Geometry check sheet. Reference: the model listing, model coordinates, mm. A direction names the side the tool comes from. Give positions to 0.01 mm unless a question says otherwise; leave off trailing zeros. Order: outer loops, then holes, each group sorted by start corner. A loop starts at its lowest first (then second) coordinate and runs counter-clockwise, first axis right, second up. Notation, with made-up numbers: M 57,33 L 94,33 A21 cw 94,56 Z; hole C -7,77.5 d11. An arc over 180 degrees is marked long. Answer as CSV lines item,"result". Start each with the question number.
```python
from build123d import *

# Parameters (mm, degrees)
RESSALTO_EXTRUS_O3_DEPTH   = 89
FILETE3_R                  = 1
ESBO_O16_W                 = 12
ESBO_O16_H                 = 1
RESSALTO_EXTRUS_O5_DEPTH   = 0.5
FILETE7_R                  = 0.5
CORTE_EXTRUS_O9_DEPTH      = 200
CORTE_EXTRUS_O9_DEPTH_BACK = 10
ESBO_O22_R                 = 1.25
ESBO_O22_W                 = 8
ESBO_O22_H                 = 15
CORTE_EXTRUS_O10_DEPTH     = 322.757399842
RESSALTO_EXTRUS_O8_DEPTH   = 2
FILETE12_R                 = 10
FILETE13_R                 = 4
ESBO_O30_W                 = 10
ESBO_O30_H                 = 1.5
RESSALTO_EXTRUS_O10_DEPTH  = 0.75
FILETE14_R                 = 0.75
RESSALTO_EXTRUS_O11_START  = -20
RESSALTO_EXTRUS_O11_DEPTH  = 5


with BuildPart() as part:
    # Esboço6 → Ressalto-extrusão3 (new body)
    with BuildSketch(Plane(origin=(0, -284.347629413, 0), x_dir=(1, 0, 0), z_dir=(0, 1, 0))):
        Polygon((4.5, 12.61291239), (2.5, 12.61291239), (2.5, 32.61291239), (149.5, 32.61291239), (149.5, 12.61291239), (147.5, 12.61291239), (147.5, 30.61291239), (4.5, 30.61291239), align=None)
    extrude(amount=RESSALTO_EXTRUS_O3_DEPTH)

    # Filete3
    filete3_edges = [part.edges().sort_by_distance(p)[0] for p in [
        (2.5, -239.847629413, -32.61291239),
        (149.5, -239.847629413, -32.61291239),
    ]]
    fillet(filete3_edges, radius=FILETE3_R)

    # Esboço16 → Ressalto-extrusão5 (add)
    with BuildSketch(Plane.XY.offset(-30.61291239)):
        with Locations((62, -266.847629413)):
            Rectangle(ESBO_O16_W, ESBO_O16_H)
    extrude(amount=RESSALTO_EXTRUS_O5_DEPTH)

    # Filete7
    filete7_edges = [part.edges().sort_by_distance(p)[0] for p in [
        (56, -266.847629413, -30.61291239),
        (68, -266.847629413, -30.61291239),
        (62, -266.347629413, -30.61291239),
        (62, -267.347629413, -30.61291239),
    ]]
    fillet(filete7_edges, radius=FILETE7_R - 0.0001)  # a hair under: the kernel refuses the full size

    # Esboço20 → Corte-extrusão9 (cut, two sides: drawn at the far end of the back side and taken through both)
    with BuildSketch(Plane.ZY.offset(-147.5).offset(-CORTE_EXTRUS_O9_DEPTH_BACK)):
        Polygon((-27.61291239, -195.347629413), (-12.61291239, -195.347629413), (-12.61291239, -248.347629413), align=None)
        with BuildLine():
            Line((-19.964933879, -248.075306948), (-24.796932275, -231.002245945))
            ThreePointArc((-24.796932275, -231.002245945), (-25.896604597, -230.284061963), (-26.759138321, -231.274568411))
            Line((-26.759138321, -231.274568411), (-26.759138321, -248.347629413))
            ThreePointArc((-26.759138321, -248.347629413), (-26.466245102, -249.054736195), (-25.759138321, -249.347629413))
            Line((-25.759138321, -249.347629413), (-20.927139924, -249.347629413))
            ThreePointArc((-20.927139924, -249.347629413), (-20.129542762, -248.950819903), (-19.964933879, -248.075306948))
        make_face()
    extrude(amount=CORTE_EXTRUS_O9_DEPTH + CORTE_EXTRUS_O9_DEPTH_BACK, mode=Mode.SUBTRACT)

    # Esboço22 → Corte-extrusão10 (cut, through all)
    with BuildSketch(Plane.XY.offset(-30.61291239)):
        with Locations((16.25, -277.347629413)):
            Circle(ESBO_O22_R)
        with Locations((135.75, -277.347629413)):
            Circle(ESBO_O22_R)
        with BuildLine():
            Line((131.970562748, -195.347629413), (20.029437252, -195.347629413))
            Line((20.029437252, -195.347629413), (67.514718626, -242.832910788))
            ThreePointArc((67.514718626, -242.832910788), (76, -246.347629413), (84.485281374, -242.832910788))
            Line((84.485281374, -242.832910788), (131.970562748, -195.347629413))
        make_face()
        with BuildLine():
            Line((134.5, -223.688249847), (134.5, -242.347629413))
            ThreePointArc((134.5, -242.347629413), (133.328427125, -245.176056538), (130.5, -246.347629413))
            Line((130.5, -246.347629413), (111.840620434, -246.347629413))
            ThreePointArc((111.840620434, -246.347629413), (108.145102304, -243.878363143), (109.012193309, -239.519202289))
            Line((109.012193309, -239.519202289), (127.671572875, -220.859822722))
            ThreePointArc((127.671572875, -220.859822722), (132.030733729, -219.992731717), (134.5, -223.688249847))
        make_face()
        with BuildLine():
            Line((17.5, -223.688249847), (17.5, -242.347629413))
            ThreePointArc((17.5, -242.347629413), (18.671572875, -245.176056538), (21.5, -246.347629413))
            Line((21.5, -246.347629413), (40.159379566, -246.347629413))
            ThreePointArc((40.159379566, -246.347629413), (43.854897696, -243.878363143), (42.987806691, -239.519202289))
            Line((42.987806691, -239.519202289), (24.328427125, -220.859822722))
            ThreePointArc((24.328427125, -220.859822722), (19.969266271, -219.992731717), (17.5, -223.688249847))
        make_face()
        with Locations((62, -276.847629413)):
            Rectangle(ESBO_O22_W, ESBO_O22_H)
    extrude(amount=-CORTE_EXTRUS_O10_DEPTH, mode=Mode.SUBTRACT)

    # Esboço25 → Ressalto-extrusão8 (add)
    with BuildSketch(Plane(origin=(0, -195.347629413, 0), x_dir=(1, 0, 0), z_dir=(0, 1, 0))):
        Polygon((147.5, 30.61291239), (142.5, 30.61291239), (147.5, 27.61291239), align=None)
        Polygon((4.5, 30.61291239), (9.5, 30.61291239), (4.5, 27.61291239), align=None)
    extrude(amount=-RESSALTO_EXTRUS_O8_DEPTH)

    # Filete12
    filete12_edges = [part.edges().sort_by_distance(p)[0] for p in [
        (20.029437252, -195.347629413, -31.61291239),
        (131.970562748, -195.347629413, -31.61291239),
    ]]
    fillet(filete12_edges, radius=FILETE12_R)

    # Filete13
    filete13_edges = [part.edges().sort_by_distance(p)[0] for p in [
        (58, -269.347629413, -31.61291239),
        (66, -269.347629413, -31.61291239),
    ]]
    fillet(filete13_edges, radius=FILETE13_R - 0.0001)  # a hair under: the kernel refuses the full size

    # Esboço30 → Ressalto-extrusão10 (add)
    with BuildSketch(Plane.XY.offset(-30.61291239)):
        with Locations((91.5, -258.597629413)):
            Rectangle(ESBO_O30_W, ESBO_O30_H)
    extrude(amount=RESSALTO_EXTRUS_O10_DEPTH)

    # Filete14
    filete14_edges = [part.edges().sort_by_distance(p)[0] for p in [
        (91.5, -257.847629413, -29.86291239),
        (91.5, -259.347629413, -29.86291239),
    ]]
    fillet(filete14_edges, radius=FILETE14_R - 0.0001)  # a hair under: the kernel refuses the full size

    # Esboço31 → Ressalto-extrusão11 (add)
    with BuildSketch(Plane.XZ.offset(284.347629413).offset(RESSALTO_EXTRUS_O11_START)):
        with BuildLine():
            Line((147.5, -30.61291239), (142.5, -30.61291239))
            ThreePointArc((142.5, -30.61291239), (146.035533906, -29.148446296), (147.5, -25.61291239))
            Line((147.5, -25.61291239), (147.5, -30.61291239))
        make_face()
        with BuildLine():
            Line((4.5, -30.61291239), (9.5, -30.61291239))
            ThreePointArc((9.5, -30.61291239), (5.964466094, -29.148446296), (4.5, -25.61291239))
            Line((4.5, -25.61291239), (4.5, -30.61291239))
        make_face()
    extrude(amount=-RESSALTO_EXTRUS_O11_DEPTH)


solid = part.part
```
Item 1: Depth check by flat-ended pin: pin 1 Ø1 at (x, y) = (148.5, -240.5) entering from +Z; pin 2 Ø2.5 at (x, z) = (7.5, -29) entering from -Y; pin 3 Ø0.6 at (x, z) = (123, -32) entering from +Y. Enter the tip coordinate at first touch or a pass-through.
Item 2: Section check B-B on z = -23.25. Record the boundary of the cut face in (x, y), then the cut area to 3 significant figures.
Item 3: Scan lines: line 1 along X through (y, z) = (-248.5, -18.25); line 2 along Y through (x, z) = (135.75, -31.4); line 3 along X through (y, z) = (-237.5, -31). Record each from-to range of solid material in increasing order.
Item 4: Draft check along X on faces 4 (the face through (148.514, -239.658, -22.347)), 5 (the face through (4.5, -250, -22)). Enter one of: pulls with the +X half, pulls with the -X half, needs draft (parallel to the pull), parting line crosses it, or undercut.
Item 5: Section check D-D on z = -15. Record the boundary of the cut face in (x, y), then the cut area to 3 significant figures.
Item 6: Access from +Z, -Z, +X, -X, +Y, -Y to the whole of each face (thin tool, end or side, straight path). Record for faces 1 (the face through (5.5, -259.348, -29.4)), 2 (the face through (131.97, -219.97, -31.6)), 3 (the face through (3.514, -239.658, -22.347)).
Item 7: Section check A-A on y = -213. Record the boundary of the cut face in (x, z).
Item 8: Section check C-C on x = 27.5. Record the boundary of the cut face in (y, z).
Numbers:
1,pin 1,"z = -14.69"
1,pin 2,"y = -264.35"
1,pin 3,"y = -204.02"
2,outline,"M 2.5,-284.35 L 4.5,-284.35 L 4.5,-249.35 L 2.5,-249.35 Z; M 2.5,-236.47 L 4.5,-236.47 L 4.5,-210.76 L 2.5,-210.76 Z; M 147.5,-284.35 L 149.5,-284.35 L 149.5,-249.35 L 147.5,-249.35 Z; M 147.5,-236.47 L 149.5,-236.47 L 149.5,-210.76 L 147.5,-210.76 Z"
2,area,"243 mm2"
3,line 1,"2.5 to 4.5, 147.5 to 149.5"
3,line 2,"-284.35 to -278.6, -276.1 to -195.35"
3,line 3,"2.5 to 17.5, 40.97 to 62.18, 89.82 to 111.03, 134.5 to 149.5"
4,face 4,"needs draft"
4,face 5,"undercut"
5,outline,"M 2.5,-284.35 L 4.5,-284.35 L 4.5,-239.91 L 2.5,-239.91 Z; M 147.5,-284.35 L 149.5,-284.35 L 149.5,-239.91 L 147.5,-239.91 Z"
5,area,"178 mm2"
6,face 1,"+Z"
6,face 2,"+Z, -Z"
6,face 3,"+X, -X"
7,outline,"M 2.5,-31.61 A1 ccw 3.5,-32.61 L 37.68,-32.61 L 37.68,-30.61 L 4.5,-30.61 L 4.5,-22.62 L 2.5,-22.62 Z; M 114.32,-32.61 L 148.5,-32.61 A1 ccw 149.5,-31.61 L 149.5,-22.62 L 147.5,-22.62 L 147.5,-30.61 L 114.32,-30.61 Z"
8,outline,"M -284.35,-32.61 L -246.35,-32.61 L -246.35,-30.61 L -284.35,-30.61 Z; M -224.03,-32.61 L -202.82,-32.61 L -202.82,-30.61 L -224.03,-30.61 Z"
